Could you check a few things on this model? Use its own coordinates, in mm. A direction names the side the tool comes from. Give positions to 0.01 mm unless a question says otherwise; leave off trailing zeros. Loops run counter-clockwise (first coordinate to the right, second up) from the corner with the lowest first, then second, coordinate; pieces in that order, holes last.
1. Imagine slicing it at B-B (z = -74). List the corners of the cut face in (x, y) for me (3 decimals).
2. Imagine slicing it at A-A (x = -6.5). List the corners of the cut face in (y, z) for me (3 decimals), plus the area to 3 significant figures.
3. Thinking about a two-plate mould opening in Y: for faces 3 (the flat face through (6.35, 6, -77)), 4 (the cylindrical face through (-26.68, 4.65, -152.62)), 5 (the cylindrical face through (-75.02, 6.06, -152.62)), 6 (the flat face through (5, 0, -111)), which applies, +Y half, -Y half, draft (parallel to the pull), parting line (faces both ways), or undercut?
4. I need wall thicknesses on line 1 along Z through (x, y) = (-10.5, 3) (3 decimals); line 2 along X through (y, z) = (2.75, -5) (3 decimals). Which ranges of each line are inside material? Lowest first, please.
5. For faces 1 (the cylindrical face through (4.44, 6.26, -152.42)), 2 (the flat face through (-39, 6, -151.054)), which set-ups out of +Z, -Z, +X, -X, +Y, -Y let a thin tool reach every point of the face, with its end or its side?
6. For P1, Ø4, axis at y = 9.5, z = -131.5, coming from the -X side (3 decimals), with a flat end and sliding along its axis, tell me the tip position at first contact or that it passes through.
Autodesk Inventor part; units mm, degrees
ref_plane "YZ Plane" through (0, 0, 0) normal (1, 0, 0) x (0, 1, 0)
ref_plane "XZ Plane" through (0, 0, 0) normal (0, 1, 0) x (-1, 0, 0)
ref_plane "XY Plane" through (0, 0, 0) normal (0, 0, 1) x (1, 0, 0)
sketch "Sketch1" plane through (0, 0, 0) normal (0, 0, 1) x (1, 0, 0)
  line L0 (0, 0) -> (-79.2226, 0)
  line L1 (-79.2226, 0) -> (-79.2226, 12.7)
  line L2 (-79.2226, 12.7) -> (0, 12.7)
  line L3 (0, 12.7) -> (0, 0)
  line L4 (0, 12.7) -> (-29.718, 12.7)
  line L5 (-79.2226, 12.7) -> (-71.7296, 12.7)
  dimension "d1" = 79.2226
  dimension "d2" = 12.7
  dimension "d5" = 7.493
extrude "Plate5" add sketch "Sketch1" along normal blind 3.175
sketch "Sketch6" plane through (3.175, 0, -3.175) normal (1, 0, 0) x (0, 1, 0)
  line L0 (12.7, 0) -> (0, 0)
  line L1 (0, 0) -> (0, -144.7038)
  line L2 (0, -144.7038) -> (12.7, -144.7038)
  line L3 (12.7, -144.7038) -> (12.7, 0)
edge flange "Flange4" height 151.0538 angle 90 thickness 3.175 bend radius 3.175 thickness toward (1, 0, 0) relief tear relief width 3.175 relief depth 1.5875 edges at (0, 6.35, 0) wall of the first edge with corners at (3.175, 12.7, -3.175) (3.175, 0, -3.175) (3.175, 0, -147.8788) (3.175, 12.7, -147.8788)
bend "Bend4"
corner "Corner4"
sketch "Sketch7" plane through (0, 0, -151.0538) normal (0, 0, -1) x (-1, 0, 0)
  line L0 (0, 12.7) -> (0, 0)
  line L1 (0, 0) -> (79.2226, 0)
  line L2 (79.2226, 0) -> (79.2226, 12.7)
  line L3 (79.2226, 12.7) -> (0, 12.7)
edge flange "Flange5" height 85.5726 angle 90 thickness 3.175 bend radius 3.175 thickness toward (0, 0, -1) relief tear relief width 3.175 relief depth 1.5875 edges at (3.175, 6.35, -147.8788) wall of the first edge with corners at (0, 12.7, -151.0538) (0, 0, -151.0538) (-79.2226, 0, -151.0538) (-79.2226, 12.7, -151.0538)
bend "Bend5"
corner "Corner5"
sketch "Sketch8" plane through (0, 0, 3.175) normal (0, 0, 1) x (1, 0, 0)
  circle A0 centre (-71.725, 5.9188) radius 3.3
  circle A1 centre (-29.725, 5.9188) radius 3.3
extrude "Extrusion2" cut sketch "Sketch8" against normal blind 2539974.6
equation "\"d43\" = BendReliefWidth"
equation "\"d44\" = BendReliefDepth"
equation "\"d45\" = MinimumRemnant"
equation "\"d46\" = BendRadius"
equation "\"d49\" = BendRadius"
equation "\"d50\" = CornerReliefSize"
equation "\"d51\" = GapSize"
equation "\"d52\" = JacobiRadiusSize"
equation "\"d53\" = BendReliefWidth"
equation "\"d54\" = BendReliefDepth"
equation "\"d55\" = MinimumRemnant"
equation "\"d56\" = BendRadius"
equation "\"d59\" = BendRadius"
equation "\"d60\" = CornerReliefSize"
equation "\"d61\" = GapSize"
equation "\"d62\" = JacobiRadiusSize"
equation "\"BendRadius\" = Thickness"
equation "\"BendReliefWidth\" = Thickness"
equation "\"BendReliefDepth\" = 0.5 * Thickness"
equation "\"CornerReliefSize\" = 4 * Thickness"
equation "\"MinimumRemnant\" = 2 * Thickness"
equation "\"TransitionRadius\" = BendRadius"
equation "\"JacobiRadiusSize\" = BendRadius"
equation "\"GapSize\" = Thickness"
equation "\"d8\" = BendRadius"
equation "\"d42\" = BendRadius"
properties part number "tie-together tier 1 wide" material "Aluminum 6061"
Derived:
1. outline: (3.175, 0) - (6.35, 0) - (6.35, 12.7) - (3.175, 12.7) - close
2. outline: (0, -154.229) - (12.7, -154.229) - (12.7, -151.054) - (0, -151.054) - close; (0, 0) - (12.7, 0) - (12.7, 3.175) - (0, 3.175) - close
2. area: 80.6 mm2
3. face 3: draft
3. face 4: undercut
3. face 5: undercut
3. face 6: -Y half
4. line 1: z = -154.229 to -151.054, 0 to 3.175
4. line 2: x = 3.175 to 6.35
5. face 1: -Z, +X, +Y, -Y
5. face 2: -X, +Y, -Y
6. P1: stops at x = 3.175
